Check sheet for the modelled part. Datum: model origin and axes. Units: mm. A direction names the side the tool comes from. Round coordinates to 2 decimals unless told otherwise and drop trailing zeros. Loops run counter-clockwise (first coordinate to the right, second up) from the corner with the lowest first, then second, coordinate; pieces in that order, holes last. Notation, with made-up numbers: (31, 53.25) -> (82, 53.25) arc R29 cw to (82, 90.25) -> close; hole circle Ø3 at (65.5, 19). An arc over 180 degrees is marked (long way). Use one line per item in the form item = value. Start each with the question number.
(1) Material ranges on probe 1 along Z at (x, y) = (125, 2.5); probe 2 along Z at (x, y) = (37, 1.75); probe 3 along Z at (x, y) = (157, 6.5), recorded low to high. Write a range as [from, to].
(2) Set-up check for faces 4 (the flat face through (17.57, 2.55, 4.29)), 5 (the cylindrical face through (126.526, 4.437, 10.481)), 6 (the flat face through (158.05, 1.43, 1.65)): record each of +Z, -Z, +X, -X, +Y, -Y from which the full face is reachable in a straight line by a thin tool's end or side.
(3) Sectioned sample at B-B (x = 34.5). Record the cut outline in (y, z), and give its area (3 significant figures).
(4) Go/stop test with flat-tipped pins: pin 1 (3 mm diameter, centred on x = 88.5, z = 10, fed in from -Y); pin 2 (3.5 mm diameter, centred on x = 15, y = 4, fed in from +Z); pin 3 (1 mm diameter, centred on y = 4.5, z = 2.5, fed in from +X). Record where each tip stops, or that it passes through.
(5) Sectioned sample at A-A (x = 147). Record the cut outline in (y, z), and give its area (4 significant figures).
(6) Sectioned sample at C-C (x = 125). Record the cut outline in (y, z), and give its area (3 significant figures).
(7) Draft check along X on faces 1 (the flat face through (96.46, 2.5, 11.52)), 2 (the flat face through (149.29, 6.437, 7.084)), 3 (the flat face through (87, 5, 13)). Enter one of: released by +X, released by -X, zero draft, split by the parting line, or undercut.
Autodesk Inventor part; units mm, degrees
ref_plane "YZ Plane" through (0, 0, 0) normal (1, 0, 0) x (0, 1, 0)
ref_plane "XZ Plane" through (0, 0, 0) normal (0, 1, 0) x (-1, 0, 0)
ref_plane "XY Plane" through (0, 0, 0) normal (0, 0, 1) x (1, 0, 0)
sketch "Sketch1" plane through (0, 0, 0) normal (0, 0, 1) x (1, 0, 0)
  line L0 (0, 0) -> (164.5, 0)
  line L1 (164.5, 0) -> (164.5, 9)
  line L2 (164.5, 9) -> (0, 9)
  line L3 (0, 9) -> (0, 0)
  circle A0 centre (99, 4) radius 1.6
  circle A1 centre (159.5, 4) radius 1.6
  circle A2 centre (147, 4) radius 1.6
  circle A3 centre (15, 4) radius 1.6
  circle A4 centre (7, 4) radius 1.6
  dimension "d1" = 9
  dimension "d2" = 90
  dimension "d6" = 3.2
  dimension "d7" = 3.2
  dimension "d9" = 60.5
  dimension "d26" = 3.2
  dimension "d27" = 48
  dimension "d28" = 3.2
  dimension "d32" = 15
  dimension "d33" = 5
  dimension "d61" = 3.2
  dimension "d62" = 8
  dimension "d63" = 12.5
  dimension "d108" = 4
  dimension "d109" = 4
  dimension "d111" = 4
  dimension "d112" = 4
  dimension "d113" = 4
ref_plane "Work Plane2" through (0, 0, 0) normal (0, -1, 0) x (1, 0, 0)
sketch "Sketch2" plane through (0, 0, 0) normal (0, -1, 0) x (1, 0, 0)
  circle A0 centre (52, 10) radius 1.6
  circle A1 centre (125, 10) radius 1.6
  circle A2 centre (88.5, 10) radius 1.6
  point P0 (0, 0)
  point P1 (52, 0)
  dimension "d13" = 3.2
  dimension "d15" = 3.2
  dimension "d17" = 3.2
  dimension "d18" = 36.5
  dimension "d64" = 52
  dimension "d65" = 36.5
  dimension "d114" = 10
  dimension "d115" = 73
ref_plane "Work Plane1" through (0, 0, 11) normal (0, 0, 1) x (1, 0, 0)
extrude "klocek" add sketch "Sketch1" along normal blind 13
ref_plane "Work Plane3" through (0, 0, 0) normal (0, -1, 0) x (1, 0, 0)
extrude "prowadzenie osi" cut sketch "Sketch2" against normal up to next
ref_plane "Work Plane4" through (0, 0, 0) normal (0, -1, 0) x (1, 0, 0)
sketch "Sketch7" plane through (0, 0, 0) normal (0, -1, 0) x (1, 0, 0)
  line L0 (0, 13) -> (0, 1)
  line L1 (0, 13) -> (164.5, 13)
  line L2 (0, 13) -> (40, 13)
  line L3 (40, 13) -> (0, 1)
  point P0 (0, -1.8333)
  dimension "d86" = 12
  dimension "d87" = 40
sketch "Sketch8" plane through (0, 0, 0) normal (0, -1, 0) x (1, 0, 0)
  line L0 (164.5, 0) -> (164.5, 13)
  line L1 (164.5, 13) -> (164.5, 1)
  line L2 (164.5, 13) -> (0, 13)
  line L3 (164.5, 13) -> (134.5, 13)
  line L4 (134.5, 13) -> (164.5, 1)
  point P0 (0, 0)
  point P1 (40.8333, 11)
  dimension "d80" = 12
  dimension "d81" = 30
extrude "przedni skos" cut sketch "Sketch7" against normal up to next
extrude "tylni skos" cut sketch "Sketch8" against normal up to next
ref_plane "Work Plane7" through (0, 0, 11) normal (0, 0, 1) x (1, 0, 0)
sketch "Sketch5" plane through (0, 0, 13) normal (0, 0, 1) x (1, 0, 0)
  circle A0 centre (99, 4) radius 1.6
  line L0 (95.5936, 4) -> (97.2968, 6.95)
  line L1 (97.2968, 6.95) -> (100.7032, 6.95)
  line L2 (100.7032, 6.95) -> (102.4064, 4)
  line L3 (102.4064, 4) -> (100.7032, 1.05)
  line L4 (100.7032, 1.05) -> (97.2968, 1.05)
  line L5 (97.2968, 1.05) -> (95.5936, 4)
  point P0 (119.5, 5)
  dimension "d98" = 5.9
extrude "hex insert middle" cut sketch "Sketch5" against normal blind 3
ref_plane "Work Plane6" through (0, 0, 11) normal (0, 0, 1) x (1, 0, 0)
sketch "Sketch9" plane through (0, 0, 11) normal (0, 0, 1) x (1, 0, 0)
  circle A0 centre (147, 4) radius 1.6
  line L0 (150.4064, 4) -> (148.7032, 1.05)
  line L1 (148.7032, 1.05) -> (145.2968, 1.05)
  line L2 (145.2968, 1.05) -> (143.5936, 4)
  line L3 (143.5936, 4) -> (145.2968, 6.95)
  line L4 (145.2968, 6.95) -> (148.7032, 6.95)
  line L5 (148.7032, 6.95) -> (150.4064, 4)
  point P0 (0, 0)
  point P1 (153, 5)
  dimension "d99" = 5.9
extrude "hex insert rear 1" cut sketch "Sketch9" against normal blind 7.5
ref_plane "Work Plane5" through (0, 0, 11) normal (0, 0, 1) x (1, 0, 0)
sketch "Sketch10" plane through (0, 0, 11) normal (0, 0, 1) x (1, 0, 0)
  circle A0 centre (159.5, 4) radius 1.6
  line L0 (162.45, 5.7032) -> (162.45, 2.2968)
  line L1 (162.45, 2.2968) -> (159.5, 0.5936)
  line L2 (159.5, 0.5936) -> (156.55, 2.2968)
  line L3 (156.55, 2.2968) -> (156.55, 5.7032)
  line L4 (156.55, 5.7032) -> (159.5, 7.4064)
  line L5 (159.5, 7.4064) -> (162.45, 5.7032)
  line L6 (164.5, 0) -> (134.5, 0)
  point P0 (0, 0)
  dimension "d118" = 5.9
extrude "hex insert rear 2" cut sketch "Sketch10" against normal up to next contours A0 | L0 L1 L2 L3 L4 L5
sketch "Sketch13" plane through (0, 0, 11) normal (0, 0, 1) x (1, 0, 0)
  circle A0 centre (7, 4) radius 1.6
  line L0 (10.4064, 4) -> (8.7032, 1.05)
  line L1 (8.7032, 1.05) -> (5.2968, 1.05)
  line L2 (5.2968, 1.05) -> (3.5936, 4)
  line L3 (3.5936, 4) -> (5.2968, 6.95)
  line L4 (5.2968, 6.95) -> (8.7032, 6.95)
  line L5 (8.7032, 6.95) -> (10.4064, 4)
  dimension "d123" = 5.9
extrude "hex insert front 1" cut sketch "Sketch13" against normal through all
sketch "Sketch16" plane through (0, 0, 11) normal (0, 0, 1) x (1, 0, 0)
  circle A0 centre (15, 4) radius 1.6
  line L0 (18.4064, 4) -> (16.7032, 1.05)
  line L1 (16.7032, 1.05) -> (13.2968, 1.05)
  line L2 (13.2968, 1.05) -> (11.5936, 4)
  line L3 (11.5936, 4) -> (13.2968, 6.95)
  line L4 (13.2968, 6.95) -> (16.7032, 6.95)
  line L5 (16.7032, 6.95) -> (18.4064, 4)
  point P0 (0, 0)
  dimension "d93" = 5.9
extrude "hex insert front 2" cut sketch "Sketch16" against normal blind 9
sketch "Sketch17" plane through (0, 0, 0) normal (0, 0, -1) x (-1, 0, 0)
  line L0 (-164.5, 9) -> (0, 9)
  line L1 (0, 0) -> (-2, 0)
  line L2 (-2, 0) -> (-2, 9)
  line L3 (-2, 9) -> (0, 9)
  line L4 (0, 9) -> (0, 0)
  dimension "d122" = 2
extrude "ciecie przod" cut sketch "Sketch17" against normal up to next
sketch "Sketch18" plane through (40, 0, 13) normal (0, -1, 0) x (1, 0, 0)
  line L0 (9.5, 0) -> (9.5, -4)
  line L1 (9.5, -4) -> (-15.5, -4)
  line L2 (-15.5, -4) -> (-15.5, 0)
  line L3 (-15.5, 0) -> (9.5, 0)
  line L4 (94.5, 0) -> (0, 0)
  circle A0 centre (12, -3) radius 1.6
  line L5 (-40, -13) -> (124.5, -13)
  point P0 (-35, -11)
  dimension "d102" = 4
  dimension "d103" = 25
  dimension "d104" = 2.5
extrude "sensor linii" cut sketch "Sketch18" against normal blind 7.3 contours L0 L1 L2 L3
properties part number "wheel_support_v5_left_narrow_with_line_sensor_2mm_higher"
Checks:
q1.probe_1 = [0, 8.4], [11.6, 13]
q1.probe_2 = [0, 9]
q1.probe_3 = [0, 4]
q2.face_4 = +Z
q2.face_5 = +Y, -Y
q2.face_6 = +Z, -Z
q3.outline = (0, 0) -> (9, 0) -> (9, 11.35) -> (7.3, 11.35) -> (7.3, 9) -> (0, 9) -> close
q3.area = 85.0 mm2
q4.pin_1 = through
q4.pin_2 = 2
q4.pin_3 = 156.55
q5.outline = (0, 0) -> (2.4, 0) -> (2.4, 3.5) -> (1.05, 3.5) -> (1.05, 8) -> (0, 8) -> close; (5.6, 0) -> (9, 0) -> (9, 8) -> (6.95, 8) -> (6.95, 3.5) -> (5.6, 3.5) -> close
q5.area = 34.25 mm2
q6.outline = (0, 0) -> (9, 0) -> (9, 8.4) -> (0, 8.4) -> close; (0, 11.6) -> (9, 11.6) -> (9, 13) -> (0, 13) -> close
q6.area = 88.2 mm2
q7.face_1 = undercut
q7.face_2 = released by +X
q7.face_3 = zero draft
